Design review of the part built by this model. Coordinates are the model's own, in mm. Face numbers are marked on the shaded views. Give positions to 0.01 mm unless a question says otherwise; leave off trailing zeros. Loops run counter-clockwise (first coordinate to the right, second up) from the corner with the lowest first, then second, coordinate; pieces in that order, holes last. Notation, with made-up numbers: M 6.25,-24 L 53.25,-24 A22 cw 53.25,14 Z; hole C 16,27 d11. An arc over 180 degrees is marked long. Answer as CSV lines item,"result".
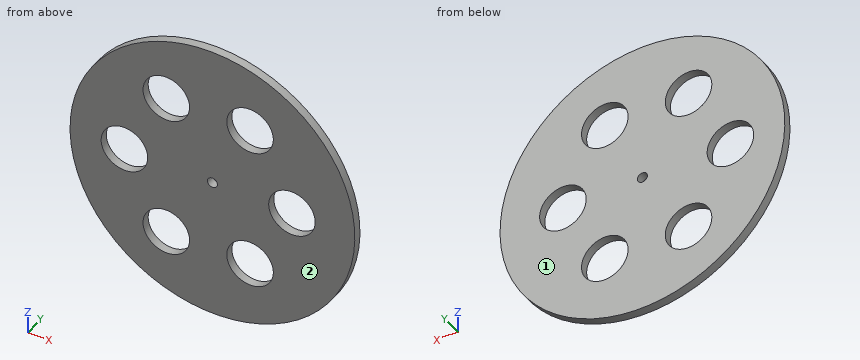
```python
from build123d import *

# Parameters (mm, degrees)
SKETCH2_R           = 85
BOSS_EXTRUDE1_DEPTH = 5
SKETCH3_R           = 13.901120553
CUT_EXTRUDE1_DEPTH  = 121.312094155
SKETCH4_R           = 3
CUT_EXTRUDE2_DEPTH  = 10


with BuildPart() as part:
    # Sketch2 → Boss-Extrude1 (new body)
    with BuildSketch(Plane(origin=(0, 0, 0), x_dir=(1, 0, 0), z_dir=(0, 1, 0))):
        with Locations(Location((0, 0, 0), (0, 0, 270))):
            Circle(SKETCH2_R)
    extrude(amount=BOSS_EXTRUDE1_DEPTH)

    # Sketch3 → Cut-Extrude1 (cut, through all)
    with BuildSketch(Plane(origin=(0, 5, 0), x_dir=(1, 0, 0), z_dir=(0, 1, 0))):
        with Locations(Location((47.468904606, 0, 0), (0, 0, 270))):
            Circle(SKETCH3_R)
        with Locations(Location((22.468904606, -43.301270189, 0), (0, 0, 270))):
            Circle(SKETCH3_R)
        with Locations(Location((-27.531095394, -43.301270189, 0), (0, 0, 270))):
            Circle(SKETCH3_R)
        with Locations(Location((-52.531095394, 0, 0), (0, 0, 270))):
            Circle(SKETCH3_R)
        with Locations(Location((-27.531095394, 43.301270189, 0), (0, 0, 270))):
            Circle(SKETCH3_R)
        with Locations(Location((22.468904606, 43.301270189, 0), (0, 0, 270))):
            Circle(SKETCH3_R)
    extrude(amount=-CUT_EXTRUDE1_DEPTH, mode=Mode.SUBTRACT)

    # Sketch4 → Cut-Extrude2 (cut)
    with BuildSketch(Plane(origin=(0, 5, 0), x_dir=(1, 0, 0), z_dir=(0, 1, 0))):
        with Locations(Location((0, 0, 0), (0, 0, 270))):
            Circle(SKETCH4_R)
    extrude(amount=-CUT_EXTRUDE2_DEPTH, mode=Mode.SUBTRACT)


solid = part.part
```
1. We need section C-C, the plane y = 3.15. Write out the cut boundary in (x, z).
Answer block:
outline,"C 0,0 d170; hole C -52.53,0 d27.8; hole C -27.53,-43.3 d27.8; hole C -27.53,43.3 d27.8; hole C 0,0 d6; hole C 22.47,-43.3 d27.8; hole C 22.47,43.3 d27.8; hole C 47.47,0 d27.8"
2. The part is to be moulded in two halves that separate along Y. For the marked faces 1 and 2, say which applies: pulls with the +Y half, pulls with the -Y half, needs draft (parallel to the pull), parting line crosses it, or undercut.
Answer block:
face 1,"pulls with the +Y half"
face 2,"pulls with the -Y half"
3. We need section A-A, the plane x = 0. Write out the cut boundary in (y, z), plus the area to 3 significant figures.
Answer block:
outline,"M 0,-85 L 5,-85 L 5,-3 L 0,-3 Z; M 0,3 L 5,3 L 5,85 L 0,85 Z"
area,"820 mm²"
4. To check wall thickness, follow L1, parallel to X at y = 2.75, z = 0; L2, parallel to X at y = 1.6, z = 36; L3, parallel to Z at x = 21.5, y = 3.1. State the ranges of each line that lie inside material, in increasing order. Write a range as [from, to].
Answer block:
L1,"[-85, -66.43], [-38.63, -3], [3, 33.57], [61.37, 85]"
L2,"[-77, -39.36], [-15.7, 10.64], [34.3, 77]"
L3,"[-82.24, -57.17], [-29.43, 29.43], [57.17, 82.24]"
5. For P1, Ø1, axis at x = -39.5, y = 3, coming from the +Z side; P2, Ø1.5, axis at x = 52, y = 2, coming from the -Z side, all flat-tipped, find the tip position at first contact; note any pin that passes through.
Answer block:
P1,"z = 75.52"
P2,"z = -67.81"
6. We need section B-B, the plane z = 0. Write out the cut boundary in (x, y).
Answer block:
outline,"M -85,0 L -66.43,0 L -66.43,5 L -85,5 Z; M -38.63,0 L -3,0 L -3,5 L -38.63,5 Z; M 3,0 L 33.57,0 L 33.57,5 L 3,5 Z; M 61.37,0 L 85,0 L 85,5 L 61.37,5 Z"
7. We need section D-D, the plane x = -47. Write out the cut boundary in (y, z), plus the area to 3 significant figures.
Answer block:
outline,"M 0,-70.82 L 5,-70.82 L 5,-12.75 L 0,-12.75 Z; M 0,12.75 L 5,12.75 L 5,70.82 L 0,70.82 Z"
area,"581 mm²"
